```python
from build123d import *

# Parameters (mm, degrees)
BOSS_EXTRUDE1_DEPTH = 1.5
CUT_EXTRUDE1_DEPTH  = 371.327819887


with BuildPart() as part:
    # Sketch1 → Boss-Extrude1 (new body)
    with BuildSketch(Plane(origin=(0, 0, 0), x_dir=(1, 0, 0), z_dir=(0, 1, 0))):
        with BuildLine():
            Line((105.927382165, 9.996293603), (158.819770869, 30.299779353))
            ThreePointArc((158.819770869, 30.299779353), (167.313965475, 30.968286967), (174.80189183, 26.902674674))
            Line((174.80189183, 26.902674674), (201.609844783, 0.094721721))
            ThreePointArc((201.609844783, 0.094721721), (207.086144351, -3.394065873), (213.523782642, -4.241597033))
            Line((213.523782642, -4.241597033), (359.215598315, 8.504785207))
            ThreePointArc((359.215598315, 8.504785207), (368.965752283, 0.323434609), (360.784401685, -9.426719358))
            Line((360.784401685, -9.426719358), (209.053654194, -22.701439672))
            ThreePointArc((209.053654194, -22.701439672), (200.470136473, -21.571398126), (193.168403715, -16.919681334))
            Line((193.168403715, -16.919681334), (172.635581566, 3.613140816))
            ThreePointArc((172.635581566, 3.613140816), (162.651679758, 9.033957206), (151.326086951, 8.142613722))
            Line((151.326086951, 8.142613722), (110.128629497, -7.67160853))
            ThreePointArc((110.128629497, -7.67160853), (106.605981016, -8.665098151), (102.961270506, -9))
            Line((102.961270506, -9), (0, -9))
            Line((0, -9), (0, 9))
            Line((0, 9), (100.551862922, 9))
            ThreePointArc((100.551862922, 9), (103.285395804, 9.251176387), (105.927382165, 9.996293603))
        make_face()
    extrude(amount=BOSS_EXTRUDE1_DEPTH)

    # Sketch2 → Cut-Extrude1 (cut, through all)
    with BuildSketch(Plane(origin=(0, 1.5, 0), x_dir=(1, 0, 0), z_dir=(0, 1, 0))):
        with BuildLine():
            Line((259.857595734, -3.199373162), (359.477065544, 5.516201113))
            ThreePointArc((359.477065544, 5.516201113), (365.977168189, 0.061967381), (360.522934456, -6.438135264))
            Line((360.522934456, -6.438135264), (260.903464647, -15.153709539))
            ThreePointArc((260.903464647, -15.153709539), (254.403362002, -9.699475807), (259.857595734, -3.199373162))
        make_face()
    extrude(amount=-CUT_EXTRUDE1_DEPTH, mode=Mode.SUBTRACT)

    # Mirror2: part across plane


with BuildPart() as part_1:
    add(part.part)
    add(part.part.mirror(Plane(origin=(0, 0, 0), x_dir=(0, 0, 1), z_dir=(1, 0, 0))))


solid = part_1.part
```
Check sheet for the modelled part. Datum: model origin and axes. Units: mm. A direction names the side the tool comes from. Coordinates: 2 decimals unless noted, no trailing zeros. Write each loop counter-clockwise with the first axis right and the second up, starting at its lowest first coordinate (ties: lowest second). Pieces come first, ordered by that corner, then holes. Notation, with made-up numbers: M -26,-32 L 6,-32 A16 ccw 6,-4 Z; hole C 36,52 d10. An arc over 180 degrees is marked long. Write item = value, one per line. Start each with the question number.
1. Thickness scan on probe 1 along Z at (x, y) = (-295.5, 1.25); probe 2 along Z at (x, y) = (61, 0.25); probe 3 along Z at (x, y) = (263.5, 0.1). Record the ranges inside material, lowest first.
2. Sectioned sample at B-B (x = 91). Record the cut outline in (y, z), then the cut area to 3 significant figures.
3. Go/stop test with flat-tipped pins: pin 1 (0.8 mm diameter, centred on x = -1.5, y = 0.5, fed in from +Z); pin 2 (4 mm diameter, centred on x = 288.5, z = 10.5, fed in from -Y). Record where each tip stops, or that it passes through.
4. Sectioned sample at A-A (y = 0.65). State how many separate pieces and enclosed holes the cut face has, then the cut area to 3 significant figures.
5. Mould release check, pull along X, two halves, no side actions. Record for faces 1 (the flat face through (285.98, 0.74, 15.97)), 2 (the flat face through (-2, 0, 0)), 3 (the flat face through (-188.018, 0.74, -13.686)): pulls with the +X half, pulls with the -X half, needs draft (parallel to the pull), parting line crosses it, or undercut.
6. Tool access check on faces 4 (the flat face through (183.05, 0.74, 6.8)), 5 (the flat face through (-2, 1.5, 0)), 6 (the flat face through (-285.35, 0.74, -2.042)). Record the directions out of +Z, -Z, +X, -X, +Y, -Y that give a thin tool (end or side, any length) a straight path to the whole face; none if there is none.
7. Sectioned sample at C-C (x = -122.5). Record the cut outline in (y, z).
The answers:
q1.probe_1 = -2.93 to 0.08, 12.13 to 15.14
q1.probe_2 = -9 to 9
q1.probe_3 = -0.13 to 2.88, 14.93 to 17.94
q2.outline = M 0,-9 L 1.5,-9 L 1.5,9 L 0,9 Z
q2.area = 27.0 mm²
q3.pin_1 = 9
q3.pin_2 = through
q4.separate_pieces = 1
q4.enclosed_holes = 2
q4.area = 11,300 mm²
q5.face_1 = pulls with the +X half
q5.face_2 = needs draft
q5.face_3 = undercut
q6.face_4 = +Z, +Y, -Y
q6.face_5 = +Z, -Z, +X, -X, +Y
q6.face_6 = -Z, +Y, -Y
q7.outline = M 0,-16.36 L 1.5,-16.36 L 1.5,2.92 L 0,2.92 Z
